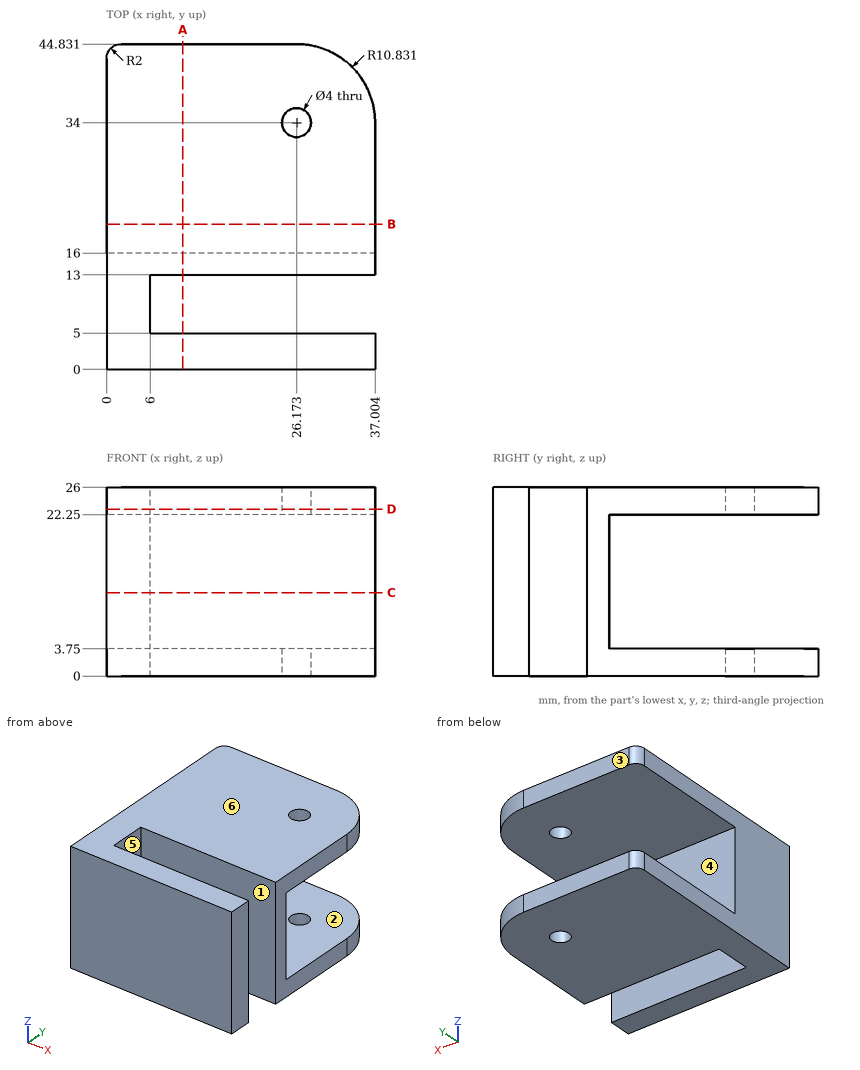
Verification items for this drawing (mm, ordinates from the low corner). A direction names the side the tool comes from. Give positions to 0.01 mm unless a question says otherwise; leave off trailing zeros. Loops run counter-clockwise (first coordinate to the right, second up) from the corner with the lowest first, then second, coordinate; pieces in that order, holes last. Notation, with made-up numbers: M 22,74 L 64,74 A23 ccw 64,86 Z; hole C 66.25,-27.75 d5. An arc over 180 degrees is marked long. Write item = value, one per line.
(1) Tool access check on the marked faces 1, 2 and 3. Record the directions out of +Z, -Z, +X, -X, +Y, -Y that give a thin tool (end or side, any length) a straight path to the whole face; none if there is none.
Answer below:
face_1 = +Z, -Z, +X
face_2 = +X, -X, +Y
face_3 = +Z, -Z, +X, -X, +Y
(2) Sectioned sample at C-C, the plane z = 11.5. Record the cut outline in (x, y), plus the area to 3 significant figures.
Answer below:
outline = M 0,0 L 37,0 L 37,5 L 6,5 L 6,13 L 37,13 L 37,16 L 0,16 Z
area = 344 mm2
(3) Sectioned sample at B-B, the plane y = 20. Record the cut outline in (x, z).
Answer below:
outline = M 0,0 L 37,0 L 37,3.75 L 0,3.75 Z; M 0,22.25 L 37,22.25 L 37,26 L 0,26 Z
(4) Sectioned sample at D-D, the plane z = 23. Record the cut outline in (x, y), plus the area to 3 significant figures.
Answer below:
outline = M 0,0 L 37,0 L 37,5 L 6,5 L 6,13 L 37,13 L 37,34 A10.83 ccw 26.17,44.83 L 2,44.83 A2 ccw 0,42.83 Z; hole C 26.17,34 d4
area = 1,370 mm2
(5) Sectioned sample at A-A, the plane x = 10.5. Record the cut outline in (y, z).
Answer below:
outline = M 0,0 L 5,0 L 5,26 L 0,26 Z; M 13,0 L 44.83,0 L 44.83,3.75 L 16,3.75 L 16,22.25 L 44.83,22.25 L 44.83,26 L 13,26 Z
(6) Gauge pin test, flat end, axial feed: pin 1 Ø12 at (x, z) = (31.5, 8.5) entering from +Y. Record the tip position at first contact, or that the pin passes through.
Answer below:
pin_1 = 44.7
(7) Release check for a two-part mould opening along Y. For the marked faces 4, 5 and 6 record: released by +Y, released by -Y, zero draft, split by the parting line, or undercut.
Answer below:
face_4 = released by +Y
face_5 = undercut
face_6 = zero draft
(8) Material ranges on line 1 (Z direction, x = 27.5, y = 23); line 2 (Y direction, x = 20.5, z = 19.5); line 3 (Y direction, x = 25, z = 23.25), recorded low to high. Write a range as [from, to].
Answer below:
line_1 = [0, 3.75], [22.25, 26]
line_2 = [0, 5], [13, 16]
line_3 = [0, 5], [13, 32.38], [35.62, 44.83]
